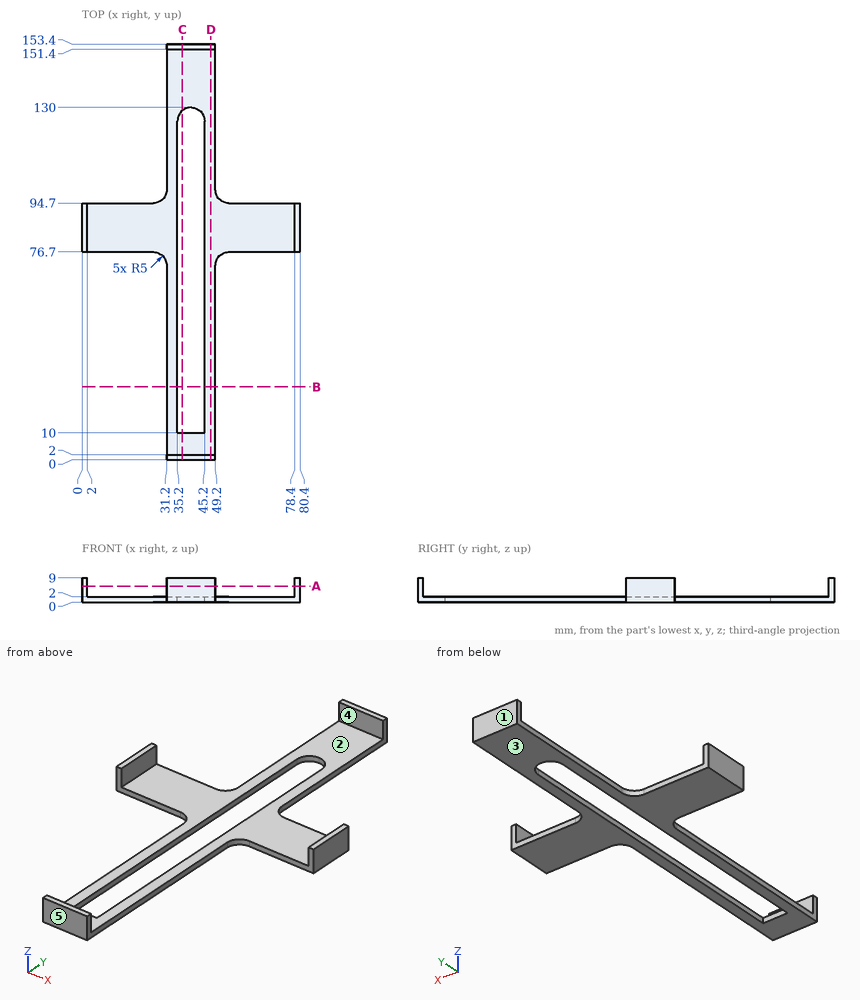
Drawing for the job (mm, zero at the part's lowest x, y, z). A direction names the side the tool comes from. Give positions to 0.01 mm unless a question says otherwise; leave off trailing zeros. Write each loop counter-clockwise with the first axis right and the second up, starting at its lowest first coordinate (ties: lowest second). Pieces come first, ordered by that corner, then holes. Notation, with made-up numbers: M -4.75,-34.75 L 6.25,-34.75 A25 ccw 6.25,-4.75 Z; hole C 62,43.5 d11. An arc over 180 degrees is marked long. Return JSON: item names as keys, results as strings. Group by question number.
(1) Band-saw the part on A-A (z = 6). Give the cut face in (x, y).
(2) Drill centre lines: L1, parallel to X at y = 19.5, z = 0.75; L2, parallel to Y at x = 48.5, z = 6; L3, parallel to X at y = 86.5, z = 8.25. Where is each one in solid material? Low to high. Write a range as [from, to].
(3) Band-saw the part on C-C (x = 37). Give the cut face in (y, z).
(4) Band-saw the part on D-D (x = 47.5). Give the cut face in (y, z), and give its area (3 significant figures).
(5) Mould opens along Y. For the marked faces 1, 2 and 3 say: pulls with the +Y half, pulls with the -Y half, needs draft (parallel to the pull), parting line crosses it, or undercut.
(6) Flat gauge pins, fed straight in: pin 1 Ø5 at (y, z) = (56, 2) entering from -X; pin 2 Ø0.6 at (y, z) = (69.5, 1.5) entering from +X; pin 3 Ø4 at (x, y) = (47, 134) entering from +Z. Where does each tip first touch, or does it go through?
(7) 3-axis set-ups, long thin cutter, end or side, ignore diameter. For the marked faces 4 and 5: which of +Z, -Z, +X, -X, +Y, -Y reach the whole face in a straight line?
(8) Band-saw the part on B-B (y = 27). Give the cut face in (x, z).
Entries:
{
 "1": {"outline": "M 0,76.7 L 2,76.7 L 2,94.7 L 0,94.7 Z; M 31.2,0 L 49.2,0 L 49.2,2 L 31.2,2 Z; M 31.2,151.4 L 49.2,151.4 L 49.2,153.4 L 31.2,153.4 Z; M 78.4,76.7 L 80.4,76.7 L 80.4,94.7 L 78.4,94.7 Z"},
 "2": {"L1": "x = [31.2, 35.2], [45.2, 49.2]", "L2": "y = [0, 2], [151.4, 153.4]", "L3": "x = [0, 2], [78.4, 80.4]"},
 "3": {"outline": "M 0,0 L 10,0 L 10,2 L 2,2 L 2,9 L 0,9 Z; M 128.84,0 L 153.4,0 L 153.4,9 L 151.4,9 L 151.4,2 L 128.84,2 Z"},
 "4": {"outline": "M 0,0 L 153.4,0 L 153.4,9 L 151.4,9 L 151.4,2 L 2,2 L 2,9 L 0,9 Z", "area": "335 mm^2"},
 "5": {"face 1": "pulls with the +Y half", "face 2": "undercut", "face 3": "needs draft"},
 "6": {"pin 1": "stops at x = 31.2", "pin 2": "stops at x = 49.2", "pin 3": "stops at z = 2"},
 "7": {"face 4": "+Z, +X, -X", "face 5": "+Z, -Z, +X, -X, -Y"},
 "8": {"outline": "M 31.2,0 L 35.2,0 L 35.2,2 L 31.2,2 Z; M 45.2,0 L 49.2,0 L 49.2,2 L 45.2,2 Z"}
}
